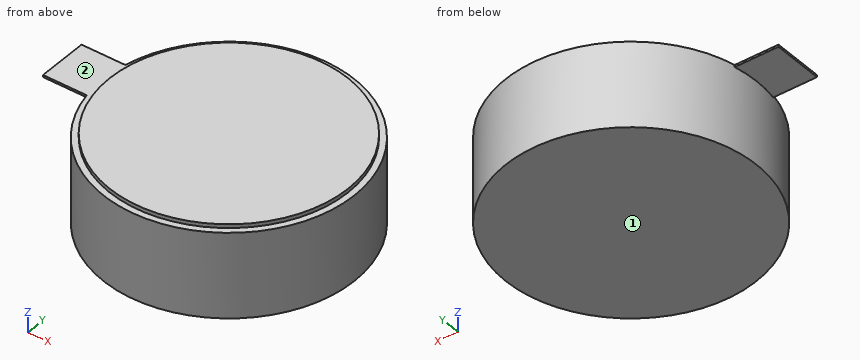
from build123d import *

# Parameters (mm, degrees)
SKETCH1_R           = 5
BOSS_EXTRUDE1_DEPTH = 3.4
SKETCH2_R           = 4.75
BOSS_EXTRUDE2_DEPTH = 0.15
BOSS_EXTRUDE3_START = -0.085
BOSS_EXTRUDE3_DEPTH = 0.085


with BuildPart() as part:
    # Sketch1 → Boss-Extrude1 (new body)
    with BuildSketch(Plane.XY):
        Circle(SKETCH1_R)
    extrude(amount=BOSS_EXTRUDE1_DEPTH)

    # Sketch2 → Boss-Extrude2 (add)
    with BuildSketch(Plane.XY.offset(3.4)):
        Circle(SKETCH2_R)
    extrude(amount=BOSS_EXTRUDE2_DEPTH)

    # Sketch4 → Boss-Extrude3 (add)
    with BuildSketch(Plane.XY.offset(3.4).offset(BOSS_EXTRUDE3_START)):
        with BuildLine():
            Line((-4.643543905, 1), (-6.643543905, 1))
            Line((-6.643543905, 1), (-6.643543905, -1))
            Line((-6.643543905, -1), (-4.643543905, -1))
            ThreePointArc((-4.643543905, -1), (-4.75, 0), (-4.643543905, 1))
        make_face()
    extrude(amount=BOSS_EXTRUDE3_DEPTH)


solid = part.part
Check sheet for the modelled part. Datum: model origin and axes. Units: mm. Face numbers are marked on the shaded views. A direction names the side the tool comes from. Round coordinates to 2 decimals unless told otherwise and drop trailing zeros. Loops run counter-clockwise (first coordinate to the right, second up) from the corner with the lowest first, then second, coordinate; pieces in that order, holes last.
1. Scan lines: probe 1 along X at (y, z) = (-0.5, 2.2); probe 2 along X at (y, z) = (3.5, 1.3); probe 3 along Y at (x, z) = (2.25, 0.9). Record each from-to range of solid material in increasing order.
2. Sectioned sample at B-B on x = -4.5. Record the boundary of the cut face in (y, z).
3. Sectioned sample at C-C on z = 2.5. Record the boundary of the cut face in (x, y).
4. Sectioned sample at D-D on y = -2.75. Record the boundary of the cut face in (x, z).
5. Set-up check for the marked faces 1 and 2: record each of +Z, -Z, +X, -X, +Y, -Y from which the full face is reachable in a straight line by a thin tool's end or side.
6. Sectioned sample at A-A on y = 0. Record the boundary of the cut face in (x, z) (3 decimals), and give its area (3 significant figures).
7. Gauge pin test, flat ends, axial feed: pin 1 Ø1.5 at (y, z) = (1, 1) entering from -X; pin 2 Ø0.5 at (x, y) = (-5.5, -0.5) entering from -Z (3 decimals). Record the tip position at first contact, or that the pin passes through.
Recorded:
1. probe 1: x = -4.97 to 4.97
1. probe 2: x = -3.57 to 3.57
1. probe 3: y = -4.47 to 4.47
2. outline: (-2.18, 0) - (2.18, 0) - (2.18, 3.4) - (1.52, 3.4) - (1.52, 3.55) - (-1.52, 3.55) - (-1.52, 3.4) - (-2.18, 3.4) - close
3. outline: circle Ø10 at (0, 0)
4. outline: (-4.18, 0) - (4.18, 0) - (4.18, 3.4) - (3.87, 3.4) - (3.87, 3.55) - (-3.87, 3.55) - (-3.87, 3.4) - (-4.18, 3.4) - close
5. face 1: -Z, +X, -X, +Y, -Y
5. face 2: +Z
6. outline: (-6.644, 3.315) - (-5, 3.315) - (-5, 0) - (5, 0) - (5, 3.4) - (4.75, 3.4) - (4.75, 3.55) - (-4.75, 3.55) - (-4.75, 3.4) - (-6.644, 3.4) - close
6. area: 35.6 mm2
7. pin 1: stops at x = -4.99
7. pin 2: stops at z = 3.315
